```python
from build123d import *

# Parameters (mm, degrees)
F0_R          = 8.5
F1_DEPTH      = 4
F3_R          = 5
F4_DEPTH      = 100
F5_W          = 4
F5_H          = 5
F9_DEPTH      = 8.501
F9_DEPTH_BACK = 25


with BuildPart() as f1:
    # F0 (on Top) → F1 (new body)
    with BuildSketch(Plane.XY):
        Circle(F0_R)
    extrude(amount=F1_DEPTH)

    # F3 (on Top) → F4 (join)
    with BuildSketch(Plane.XY):
        Circle(F3_R)
    extrude(amount=F4_DEPTH)

    # F5 (on Right) → F6 (revolve)
    with BuildSketch(Plane.YZ):
        with Locations((2, 102.5)):
            Rectangle(F5_W, F5_H)
    revolve(axis=Axis((0, 0, 102.5), (0, 0, -1)))

    # F8 (on Right) → F9 (cut, two sides)
    with BuildSketch(Plane.YZ) as f9_sk:
        Polygon((0, 106), (-5, 106), (-5, 101), align=None)
    extrude(amount=-F9_DEPTH, mode=Mode.SUBTRACT)
    extrude(f9_sk.sketch, amount=F9_DEPTH_BACK, mode=Mode.SUBTRACT)


solid = f1.part
```
Part model, mm, in its own coordinate system. A direction names the side the tool comes from. Give positions to 0.01 mm unless a question says otherwise; leave off trailing zeros. Order: outer loops, then holes, each group sorted by start corner. A loop starts at its lowest first (then second) coordinate and runs counter-clockwise, first axis right, second up. Notation, with made-up numbers: (83, 77) - (100, 77) arc R26 ccw to (100, 102) - close; hole circle Ø1 at (39.5, 57.25). An arc over 180 degrees is marked (long way). Use one line per item in the form item = value.
Item 1: Which spindle directions (+Z, -Z, +X, -X, +Y, -Y) get a long thin tool onto all of the face, cutting with end or side? Do faces 1 (the face through (-1.08, -4.88, 51.33)), 2 (the face through (0, 0, 0)). Say none if no direction does.
Solution:
face_1 = +Z
face_2 = -Z, +X, -X, +Y, -Y
Item 2: Slice it at D-D on y = 7. Give the cut face in (x, z).
Solution:
outline = (-4.82, 0) - (4.82, 0) - (4.82, 4) - (-4.82, 4) - close
Item 3: Slice it at A-A on y = 0. Give the cut face in (x, z), and give its area (3 significant figures).
Solution:
outline = (-8.5, 0) - (8.5, 0) - (8.5, 4) - (5, 4) - (5, 100) - (4, 100) - (4, 105) - (-4, 105) - (-4, 100) - (-5, 100) - (-5, 4) - (-8.5, 4) - close
area = 1,070 mm2
Item 4: Pin check, flat tips, straight feed: pin 1 Ø6 at (x, z) = (-1.5, 87.5) entering from +Y; pin 2 Ø3 at (x, y) = (5, 5) entering from +Z; pin 3 Ø10 at (x, z) = (-4.5, 53.5) entering from -Y; pin 4 Ø1.5 at (x, z) = (6, 45) entering from +Y. Stop position of each tip, or through.
Solution:
pin_1 = 5
pin_2 = 4
pin_3 = -5
pin_4 = through
Item 5: Slice it at C-C on z = 53. Give the cut face in (x, y), and give its area (3 significant figures).
Solution:
outline = circle Ø10 at (0, 0)
area = 78.5 mm2
Item 6: Probe probe 1 along Z at (x, y) = (7.5, 1.5); probe 2 along Y at (x, z) = (3, 41); probe 3 along X at (y, z) = (1, 90). List the from-to ranges inside material, lowest first. Write a range as from..to.
Solution:
probe_1 = 0..4
probe_2 = -4..4
probe_3 = -4.9..4.9
Item 7: Slice it at B-B on x = 0. Give the cut face in (y, z).
Solution:
outline = (-8.5, 0) - (8.5, 0) - (8.5, 4) - (5, 4) - (5, 100) - (4, 100) - (4, 105) - (-1, 105) - (-4, 102) - (-4, 100) - (-5, 100) - (-5, 4) - (-8.5, 4) - close
